Could you check a few things on this model? Use its own coordinates, in mm. Face numbers are marked on the shaded views. A direction names the side the tool comes from. Round coordinates to 2 decimals unless told otherwise and drop trailing zeros. Loops run counter-clockwise (first coordinate to the right, second up) from the corner with the lowest first, then second, coordinate; pieces in that order, holes last.
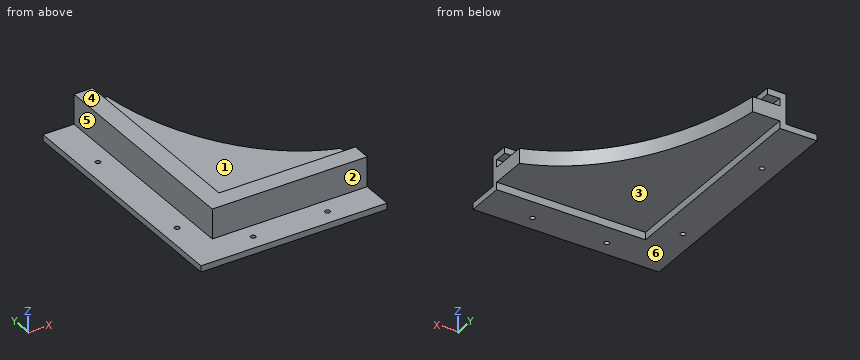
from build123d import *

# Parameters (mm, degrees)
F1_DEPTH  = 12
F2_W      = 150
F2_H      = 24
F3_DEPTH  = 5
F4_W      = 205
F4_H      = 24
F5_DEPTH  = 5
F6_R      = 2
F7_DEPTH  = 5
F9_DEPTH  = 5
F10_W     = 30
F10_H     = 30
F10_W_2   = 150
F10_H_2   = 200
F11_DEPTH = 25


with BuildPart() as f1:
    # F0 (on Top) → F1 (new body)
    with BuildSketch(Plane.XY):
        with BuildLine():
            add(Edge.make_bspline(
                [(-130, 0), (-130, -176), (0, -176)],
                knots=[1.5707963268, 1.5707963268, 1.5707963268, 3.1415926536, 3.1415926536, 3.1415926536], degree=2, weights=[1, 0.7071067812, 1]))
            Line((-130, 0), (-130, -176))
            Line((-130, -176), (0, -176))
        make_face()
        Polygon((-130, -176), (-130, 0), (-150, 0), (-150, -200), (0, -200), (0, -176), align=None)
    extrude(amount=F1_DEPTH)

    # F2 (on face) → F3 (join)
    with BuildSketch(Plane.XZ.offset(200)):
        with Locations((-75, 6)):
            Rectangle(F2_W, F2_H)
    extrude(amount=F3_DEPTH)

    # F4 (on face) → F5 (join)
    with BuildSketch(Plane(origin=(-150, 0, 0), x_dir=(0, -1, 0), z_dir=(-1, 0, 0))):
        with Locations((102.5, 6)):
            Rectangle(F4_W, F4_H)
    extrude(amount=F5_DEPTH)

    # F6 (on face) → F7 (join)
    with BuildSketch(Plane(origin=(0, 0, -6), x_dir=(1, 0, 0), z_dir=(0, 0, -1))):
        Polygon((0, 205), (0, 230), (-180, 230), (-180, 0), (-155, 0), (-155, 205), align=None)
        with Locations((-167.5, 80)):
            Circle(F6_R, mode=Mode.SUBTRACT)
        with Locations((-167.5, 180)):
            Circle(F6_R, mode=Mode.SUBTRACT)
        with Locations((-130, 217.5)):
            Circle(F6_R, mode=Mode.SUBTRACT)
        with Locations((-70, 217.5)):
            Circle(F6_R, mode=Mode.SUBTRACT)
    extrude(amount=-F7_DEPTH)

    # F8 (on face) → F9 (join)
    with BuildSketch(Plane.XY.offset(18)):
        Polygon((-140, 0), (-155, 0), (-155, -205), (0, -205), (0, -190), (-140, -190), align=None)
    extrude(amount=F9_DEPTH)

    # F10 (on Top) → F11 (cut, symmetric)
    with BuildSketch(Plane.XY):
        with Locations((-15, -15)):
            Rectangle(F10_W, F10_H)
        with Locations((-105, -15)):
            Rectangle(F10_W_2, F10_H)
        with Locations((-15, -130)):
            Rectangle(F10_W, F10_H_2)
    extrude(amount=F11_DEPTH, both=True, mode=Mode.SUBTRACT)


solid = f1.part
Item 1: For the marked faces 5 and 6, which set-ups out of +Z, -Z, +X, -X, +Y, -Y let a thin tool reach every point of the face, with its end or its side?
Results list:
face 5: +Z, -X, +Y, -Y
face 6: -Z, +X, -X, +Y, -Y
Item 2: If we section it at A-A, the plane x = -145: Please give me the cut outline in (y, z), then the cut area to 3 significant figures.
Results list:
outline: (-230, -6) - (-200, -6) - (-200, 0) - (-30, 0) - (-30, 12) - (-200, 12) - (-200, 18) - (-30, 18) - (-30, 23) - (-205, 23) - (-205, -1) - (-230, -1) - close
area: 3,160 mm2
Item 3: Will these pins go through, and if not, where does the flat tip stop? pin 1 (1.8 mm diameter, centred on x = -116, z = 16, fed in from +Y); pin 2 (3 mm diameter, centred on y = -174.5, z = 5.5, fed in from -X); pin 3 (3 mm diameter, centred on x = -124.5, y = -198, fed in from -Z).
Results list:
pin 1: stops at y = -200
pin 2: stops at x = -155
pin 3: stops at z = 0
Item 4: If I drill on line 1 along X through (y, z) = (-217.5, -4.3); line 2 along Y through (x, z) = (-167.5, -4.35); line 3 along X through (y, z) = (-180, -4.55), over which ranges is the centre line in solid material (lowest first)?
Results list:
line 1: x = -180 to -132, -128 to -72, -68 to -30
line 2: y = -230 to -182, -178 to -82, -78 to -30
line 3: x = -180 to -169.5, -165.5 to -150
Item 5: We'd pull the mould along Z, two halves only. Please class the marked faces 1, 2, 3 and 4: released by +Z, released by -Z, zero draft, split by the parting line, or undercut.
Results list:
face 1: undercut
face 2: zero draft
face 3: released by -Z
face 4: released by +Z
